Can you work these out from the model? Positions are in its coordinate system, mm. A direction names the side the tool comes from. Round coordinates to 2 decimals unless told otherwise and drop trailing zeros. Loops run counter-clockwise (first coordinate to the right, second up) from the corner with the lowest first, then second, coordinate; pieces in that order, holes last. Notation, with made-up numbers: (-35, 58) -> (4, 58) arc R24 cw to (4, 80) -> close; hole circle Ø1 at (-31, 22.5). An arc over 180 degrees is marked (long way). Use a Markdown table: item, result.
Autodesk Inventor part; units mm, degrees
ref_plane "YZ Plane" through (0, 0, 0) normal (1, 0, 0) x (0, 1, 0)
ref_plane "XZ Plane" through (0, 0, 0) normal (0, 1, 0) x (-1, 0, 0)
ref_plane "XY Plane" through (0, 0, 0) normal (0, 0, 1) x (1, 0, 0)
sketch "Sketch1" plane through (0, 0, 0) normal (0, 1, 0) x (-1, 0, 0)
  line L0 (-3.6662, 6.35) -> (3.6662, 6.35)
  line L1 (3.6662, 6.35) -> (7.3323, 0)
  line L2 (7.3323, 0) -> (3.6662, -6.35)
  line L3 (3.6662, -6.35) -> (-3.6662, -6.35)
  line L4 (-3.6662, -6.35) -> (-7.3323, 0)
  line L5 (-7.3323, 0) -> (-3.6662, 6.35)
  point P0 (0, 0)
  point P1 (0, 0)
  dimension "d0" = 12.7
extrude "Extrusion1" add sketch "Sketch1" along normal blind 55.88
sketch "Sketch2" plane through (0, 55.88, 0) normal (0, 1, 0) x (1, 0, 0)
  circle A0 centre (0, 0) radius 2.54
  dimension "d3" = 5.08
extrude "Extrusion2" cut sketch "Sketch2" against normal blind 25.4
thread "Thread1"
sketch "Sketch3" plane through (0, 0, 0) normal (0, -1, 0) x (1, 0, 0)
  circle A0 centre (0, 0) radius 2.54
  dimension "d8" = 5.08
extrude "Extrusion3" cut sketch "Sketch3" against normal blind 25.4
thread "Thread2"
properties part number "OUTK_016_Shaft3" material "Aluminum 6061"
1. I want a section at A-A (y = 11). Please give me the cut outline in (x, z), plus the area to 3 significant figures.
Answer sheet:
| item | result |
|---|---|
| outline | (-7.33, 0) -> (-3.67, -6.35) -> (3.67, -6.35) -> (7.33, 0) -> (3.67, 6.35) -> (-3.67, 6.35) -> close; hole circle Ø5.08 at (0, 0) |
| area | 119 mm² |
2. I need wall thicknesses on line 1 (Z direction, x = 0, y = 38.75); line 2 (X direction, y = 47.25, z = 0); line 3 (Y direction, x = 1.5, z = 0). Which ranges of each line are inside material? Lowest first, please.
Answer sheet:
| item | result |
|---|---|
| line 1 | z = -6.35 to -2.54, 2.54 to 6.35 |
| line 2 | x = -7.33 to -2.54, 2.54 to 7.33 |
| line 3 | y = 25.4 to 30.48 |
3. I want a section at B-B (x = 0). Please give me the cut outline in (y, z), plus the area to 3 significant figures.
Answer sheet:
| item | result |
|---|---|
| outline | (0, -6.35) -> (55.88, -6.35) -> (55.88, -2.54) -> (30.48, -2.54) -> (30.48, 2.54) -> (55.88, 2.54) -> (55.88, 6.35) -> (0, 6.35) -> (0, 2.54) -> (25.4, 2.54) -> (25.4, -2.54) -> (0, -2.54) -> close |
| area | 452 mm² |
4. If we mould it in two halves opening along X, with no side actions, what happens to faces 4 (the flat face through (-3, 55.88, 0)), 5 (the cylindrical face through (-0.33, 12.52, 2.52)), 6 (the flat face through (5.525, 27.549, 3.131))? For each: +X half, -X half, draft (parallel to the pull), parting line (faces both ways), or undercut.
Answer sheet:
| item | result |
|---|---|
| face 4 | draft |
| face 5 | undercut |
| face 6 | +X half |
5. Which directions (+Z, -Z, +X, -X, +Y, -Y) give clear straight access to the entire face, cutting with the end or side of a thin tool? Please do faces 1 (the flat face through (0, 25.4, 0)), 2 (the flat face through (0, 28, 6.35)), 3 (the cylindrical face through (-0.33, 43.36, -2.52)).
Answer sheet:
| item | result |
|---|---|
| face 1 | -Y |
| face 2 | +Z, +X, -X, +Y, -Y |
| face 3 | +Y |
6. Will these pins go through, and if not, where does the flat tip stop? pin 1 Ø3 at (y, z) = (30, 1) entering from +X; pin 2 Ø4 at (x, z) = (0, 0) entering from -Y; pin 3 Ø1 at (x, y) = (4, 10) entering from +Z; pin 4 Ø6 at (y, z) = (30.5, -4) entering from +X.
Answer sheet:
| item | result |
|---|---|
| pin 1 | stops at x = 7.33 |
| pin 2 | stops at y = 25.4 |
| pin 3 | stops at z = 6.35 |
| pin 4 | stops at x = 6.75 |
7. I want a section at C-C (z = 1.5). Please give me the cut outline in (x, y).
Answer sheet:
| item | result |
|---|---|
| outline | (-6.47, 0) -> (-2.05, 0) -> (-2.05, 25.4) -> (2.05, 25.4) -> (2.05, 0) -> (6.47, 0) -> (6.47, 55.88) -> (2.05, 55.88) -> (2.05, 30.48) -> (-2.05, 30.48) -> (-2.05, 55.88) -> (-6.47, 55.88) -> close |
8. I want a section at D-D (z = -3.75). Please give me the cut outline in (x, y).
Answer sheet:
| item | result |
|---|---|
| outline | (-5.17, 0) -> (5.17, 0) -> (5.17, 55.88) -> (-5.17, 55.88) -> close |
